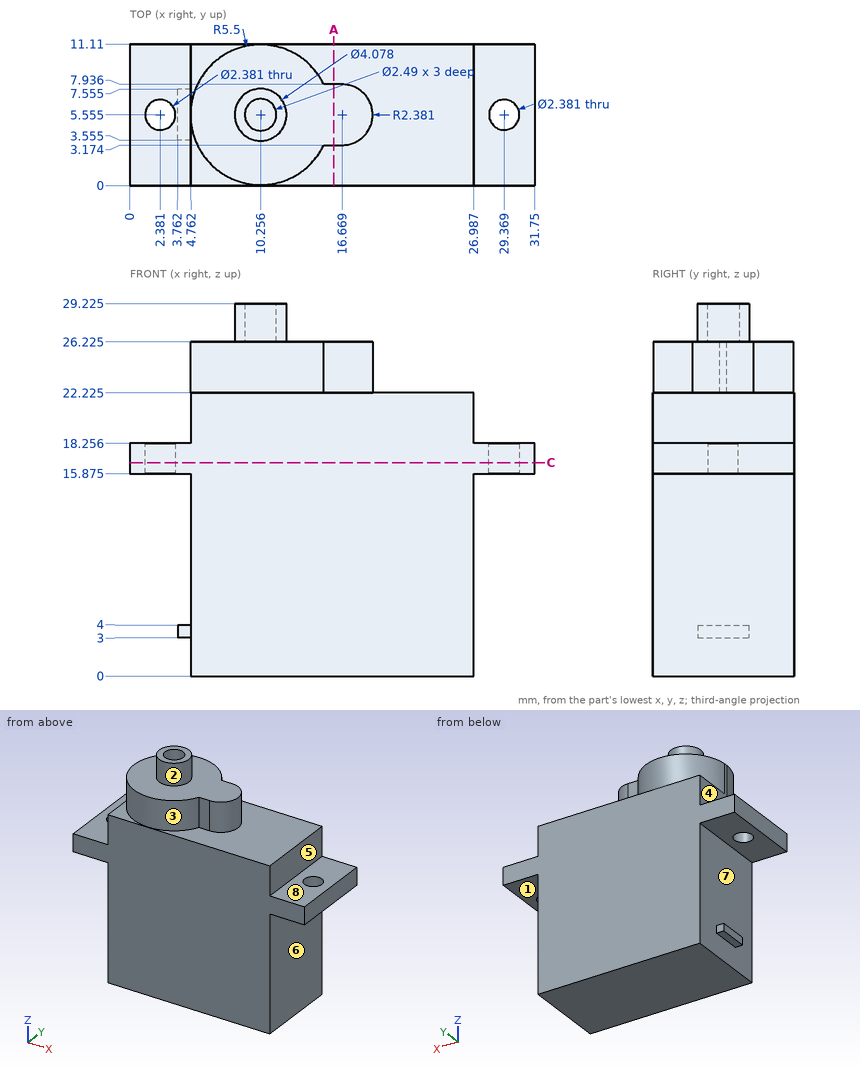
Here's the drawing with two shaded views (mm, measured from the low corner). I have some questions. A direction names the side the tool comes from. Coordinates: 2 decimals unless noted, no trailing zeros. Loops run counter-clockwise (first coordinate to the right, second up) from the corner with the lowest first, then second, coordinate; pieces in that order, holes last. Notation, with made-up numbers: M 14,73.25 L 57,73.25 A6 cw 57,80.25 Z; hole C 27,71 d8. An arc over 180 degrees is marked long. Answer as CSV lines item,"result". Start each with the question number.
1. Suppose I cut it at A-A, the plane x = 16. List the corners of the cut face in (y, z) for me (1 decimal).
2. Suppose I cut it at C-C, the plane z = 16.75. Count the separate pieces of the cut face and the enclosed holes in it, plus the area to 3 significant figures.
3. For the marked faces 1, 2, 3, 4 and 5, which set-ups out of +Z, -Z, +X, -X, +Y, -Y let a thin tool reach every point of the face, with its end or its side?
4. Thinking about a two-plate mould opening in Z: for the marked faces 6, 7 and 8, which applies, +Z half, -Z half, draft (parallel to the pull), parting line (faces both ways), or undercut?
5. If I drill on probe 1 along X at (y, z) = (5.5, 16); probe 2 along Z at (x, y) = (4.5, 3.5) (1 decimal); probe 3 along X at (y, z) = (9.25, 13.75), over which ranges is the centre line in solid material (lowest first)? Write a range as [from, to].
6. For pin 1 Ø0.7 at (x, z) = (16, 24) entering from -Y; pin 2 Ø3.5 at (y, z) = (4.5, 10) entering from -X; pin 3 Ø4 at (x, y) = (29.5, 8) entering from -Z (1 decimal), each with a flat end and sliding along its axis, tell me the tip position at first contact or that it passes through.
Output:
1,outline,"M 0,0 L 11.1,0 L 11.1,22.2 L 7.9,22.2 L 7.9,26.2 L 3.2,26.2 L 3.2,22.2 L 0,22.2 Z"
2,separate pieces,"1"
2,enclosed holes,"2"
2,area,"344 mm^2"
3,face 1,"-Z, +X, +Y, -Y"
3,face 2,"+Z"
3,face 3,"+Z, -Y"
3,face 4,"+Z, -X, +Y, -Y"
3,face 5,"+Z, +X, +Y, -Y"
4,face 6,"draft"
4,face 7,"undercut"
4,face 8,"+Z half"
5,probe 1,"x = [0, 1.19], [3.57, 28.18], [30.56, 31.75]"
5,probe 2,"z = [15.9, 18.3]"
5,probe 3,"x = [4.76, 26.99]"
6,pin 1,"stops at y = 3.17"
6,pin 2,"stops at x = 4.76"
6,pin 3,"stops at z = 15.9"
